from build123d import *

# Parameters (mm, degrees)
F1_DEPTH = 16
F2_W     = 47
F2_H     = 79.1
F3_DEPTH = 14.5
F4_W     = 5.75
F4_H     = 9.4
F5_DEPTH = 4.5
F7_DEPTH = 50.001
F9_DEPTH = 48.5


with BuildPart() as f1:
    # F0 (on Top) → F1 (new body)
    with BuildSketch(Plane.XY):
        with BuildLine():
            Line((0, 90), (0, 0))
            Line((0, 0), (50, 0))
            Line((50, 0), (50, 90))
            Line((50, 90), (34, 90))
            Line((34, 90), (34, 80))
            ThreePointArc((34, 80), (29, 75), (24, 80))
            Line((24, 80), (24, 90))
            Line((24, 90), (0, 90))
        make_face()
    extrude(amount=F1_DEPTH)

    # F2 (on face) → F3 (cut, through all)
    with BuildSketch(Plane.XY.offset(16)):
        with Locations((25, 48.95)):
            Rectangle(F2_W, F2_H)
    extrude(amount=-F3_DEPTH, mode=Mode.SUBTRACT)

    # F4 (on face) → F5 (cut)
    with BuildSketch(Plane.XY.offset(16)):
        with Locations((45.125, 4.7)):
            Rectangle(F4_W, F4_H)
        with Locations((35.375, 4.7)):
            Rectangle(F4_W, F4_H)
        with Locations((25.625, 4.7)):
            Rectangle(F4_W, F4_H)
        with Locations((15.875, 4.7)):
            Rectangle(F4_W, F4_H)
        with Locations((6.125, 4.7)):
            Rectangle(F4_W, F4_H)
    extrude(amount=-F5_DEPTH, mode=Mode.SUBTRACT)

    # F6 (on face) → F7 (cut, through all)
    with BuildSketch(Plane.YZ.offset(50)):
        Polygon((0, 8), (0, 0), (42, 0), (34, 8), align=None)
    extrude(amount=-F7_DEPTH, mode=Mode.SUBTRACT)

    # F8 (on face) → F9 (join, through all)
    with BuildSketch(Plane(origin=(0, 0, 0), x_dir=(0, -1, 0), z_dir=(-1, 0, 0))):
        Polygon((-42, 0), (-34, 8), (0, 8), (0, 9.5), (-34.6213203436, 9.5), (-44.1213203436, 0), align=None)
    extrude(amount=-F9_DEPTH)


solid = f1.part
Model file for the job. Use its own axes, mm. A direction names the side the tool comes from. Coordinates: 2 decimals unless noted, no trailing zeros. Order: outer loops, then holes, each group sorted by start corner. A loop starts at its lowest first (then second) coordinate and runs counter-clockwise, first axis right, second up. Notation, with made-up numbers: M 27,-22 L 49,-22 A25 ccw 49,-5 Z; hole C 0.5,-2.5 d9. An arc over 180 degrees is marked long. Return JSON: item names as keys, results as strings.
1. Saw through at A-A (x = 46.5). Give the cut face in (y, z), and give its area (3 significant figures).
Ans:
{"outline": "M 0,8 L 34,8 L 42,0 L 90,0 L 90,16 L 88.5,16 L 88.5,1.5 L 42.62,1.5 L 34.62,9.5 L 9.4,9.5 L 9.4,11.5 L 0,11.5 Z", "area": "181 mm^2"}
2. Drill centre lines: probe 1 along X at (y, z) = (73.5, 2.25); probe 2 along Y at (x, z) = (3, 11.25); probe 3 along Z at (x, y) = (8, 11). Where is each one in solid material? Low to high.
Ans:
{"probe 1": "0 to 1.5, 48.5 to 50", "probe 2": "0 to 9.4, 88.5 to 90", "probe 3": "8 to 9.5"}
3. Saw through at D-D (x = 25). Give the cut face in (y, z), and give its area (3 significant figures).
Ans:
{"outline": "M 0,8 L 34,8 L 42,0 L 77,0 L 77,1.5 L 42.62,1.5 L 34.62,9.5 L 9.4,9.5 L 9.4,11.5 L 0,11.5 Z", "area": "139 mm^2"}
4. Saw through at C-C (z = 5.25). Give the cut face in (x, y), and give its area (3 significant figures).
Ans:
{"outline": "M 0,36.75 L 50,36.75 L 50,90 L 34,90 L 34,88.5 L 48.5,88.5 L 48.5,38.87 L 1.5,38.87 L 1.5,88.5 L 24,88.5 L 24,90 L 0,90 Z", "area": "315 mm^2"}
5. Saw through at B-B (y = 12). Give the cut face in (x, z).
Ans:
{"outline": "M 0,8 L 50,8 L 50,16 L 48.5,16 L 48.5,9.5 L 1.5,9.5 L 1.5,16 L 0,16 Z"}
6. Tool access for faces 1 (the face through (41, 88.5, 9)), 2 (the face through (28.5, 5, 14)), 3 (the face through (9, 5, 14)): list every direction of +Z, -Z, +X, -X, +Y, -Y with a clear straight run to the whole face (end or side of a thin tool).
Ans:
{"face 1": "+Z", "face 2": "+Z, +Y, -Y", "face 3": "+Z, -Y"}
7. Flat gauge pins, fed straight in: pin 1 (1.5 mm diameter, centred on x = 9.5, z = 3, fed in from -Y); pin 2 (5 mm diameter, centred on y = 50, z = 11.5, fed in from -X); pin 3 (4.5 mm diameter, centred on x = 45, y = 6.5, fed in from +Z); pin 4 (4 mm diameter, centred on x = 39.5, y = 41, fed in from +Z). Where does each tip first touch, or does it go through?
Ans:
{"pin 1": "y = 38.25", "pin 2": "x = 0", "pin 3": "z = 11.5", "pin 4": "z = 5.12"}
8. Pull direction Y, two halves, no side cores. Call faces 4 (the face through (25, 17, 8)), 5 (the face through (29, 75, 1)), 6 (the face through (24.671, 38.565, 5.556)): +Y half, -Y half, draft (parallel to the pull), parting line (faces both ways), or undercut.
Ans:
{"face 4": "draft", "face 5": "+Y half", "face 6": "undercut"}
